Autodesk Inventor part; units mm, degrees
ref_plane "Work Plane1" through (-36, 60, 19) normal (0, -1, 0) x (1, 0, 0)
ref_plane "YZ Plane" through (0, 0, 0) normal (1, 0, 0) x (0, 1, 0)
ref_plane "XZ Plane" through (0, 0, 0) normal (0, 1, 0) x (-1, 0, 0)
sketch "Sketch1" plane through (0, 0, 0) normal (0, 0, 1) x (1, 0, 0)
  arc A0 (36, 0) -> (-36, 0) centre (0, 0) ccw
  arc A1 (27, 0) -> (-27, 0) centre (0, 0) ccw
  line L0 (-36, 0) -> (-27, 0)
  line L1 (27, 0) -> (36, 0)
  dimension "d0" = 72
  dimension "d1" = 54
  dimension "d2" = 27
  dimension "d3" = 36
extrude "Extrusion1" add sketch "Sketch1" along normal mid plane 38
ref_plane "Work Plane1" through (-36, 60, 19) normal (0, -1, 0) x (1, 0, 0)
sketch "Sketch2" plane through (-36, 60, 19) normal (0, -1, 0) x (1, 0, 0)
  line L0 (9, 0) -> (63, 0)
  line L1 (0, -38) -> (0, 0)
  line L2 (-2, -19) -> (74, -19) construction
  line L3 (-2, -31) -> (74, -31)
  line L4 (74, -7) -> (-2, -7)
  arc A0 (-2, -7) -> (-2, -31) centre (-2, -19) ccw
  arc A1 (74, -31) -> (74, -7) centre (74, -19) ccw
  point P0 (36, -19)
  point P1 (36, -19)
  point P2 (36, 0)
  point P3 (-14, -19)
  point P4 (0, -19)
  dimension "d7" = 76
  dimension "d8" = 12
extrude "Extrusion2" add sketch "Sketch2" along normal up to surface (60 mm away)
sketch "Sketch3" plane through (0, 0, 12) normal (0, 0, 1) x (1, 0, 0)
  arc A0 (27, 0) -> (-27, 0) centre (0, 0) ccw
  line L0 (-27, 0) -> (27, 0)
extrude "Extrusion3" cut sketch "Sketch3" against normal through all
sketch "Sketch4" plane through (0, 0, 0) normal (0, 0, 1) x (1, 0, 0)
  arc A0 (27, 0) -> (-27, 0) centre (0, 0) ccw
  line L0 (38, 60) -> (-38, 60)
  line L1 (-50, 60) -> (-50, 0)
  line L2 (-50, 60) -> (-50, 0)
  line L3 (-50, 60) -> (-38, 60)
  line L4 (-50, 40) -> (-24.8, 60)
  line L5 (-50, 40) -> (-50, 60)
  line L6 (0, 0) -> (0, 60) construction
  line L7 (-38, 60) -> (38, 60)
  line L8 (50, 60) -> (50, 0)
  line L9 (50, 60) -> (38, 60)
  line L10 (50, 40) -> (24.8, 60)
  point P0 (24.8, 60)
  point P1 (50, 40)
  point P2 (-50, 40)
  dimension "d13" = 20
  dimension "d14" = 25.2
extrude "Extrusion4" cut sketch "Sketch4" along normal through all both and the other way through all
fillet "Fillet1" radius 10 2 edges at (24.8, 60, 0) (-24.8, 60, 0)
sketch "Sketch5" plane through (-36, 0, 19) normal (0, -1, 0) x (1, 0, 0)
  arc A0 (-2, -7) -> (-2, -31) centre (-2, -19) ccw
  point P0 (36, -19)
  point P1 (0, -31)
  point P2 (0, -7)
hole "Hole1" at (-38, 0, 0) direction (0, 1, 0) diameter 10 end through all
sketch "Sketch6" plane through (27, 0, -19) normal (0, -1, 0) x (1, 0, 0)
  arc A0 (11, 7) -> (11, 31) centre (11, 19) ccw
  point P0 (-27, 19)
  point P1 (9, 31)
  point P2 (9, 7)
hole "Hole2" at (38, 0, 0) direction (0, 1, 0) diameter 10 end through all
sketch "Sketch7" plane through (-36, 60, 19) normal (0, 1, 0) x (1, 0, 0)
  circle A0 centre (-2, 19) radius 5
  circle A1 centre (74, 19) radius 5
  point P0 (36, 19)
hole "Hole3" at (-38, 60, 0) at (38, 60, 0) direction (0, -1, 0) diameter 10 end through all counterbore diameter 19 counterbore depth 25
fillet "Fillet2" radius 3 2 edges at (0, 36, -12) (0, 36, 12)
equation "\"d23\" = Thickness"
equation "\"BendRadius\" = Thickness"
equation "\"BendReliefWidth\" = Thickness"
equation "\"BendReliefDepth\" = 0.5 * Thickness"
equation "\"CornerReliefSize\" = 4 * Thickness"
equation "\"MinimumRemnant\" = 2 * Thickness"
equation "\"TransitionRadius\" = BendRadius"
equation "\"JacobiRadiusSize\" = BendRadius"
equation "\"GapSize\" = Thickness"
properties part number "Part 4 Connecting rods cap" material "Stainless Steel"
Geometry check sheet. Reference: the model listing, model coordinates, mm. A direction names the side the tool comes from. Give positions to 0.01 mm unless a question says otherwise; leave off trailing zeros. Loops run counter-clockwise (first coordinate to the right, second up) from the corner with the lowest first, then second, coordinate; pieces in that order, holes last. Notation, with made-up numbers: M 4,5 L 58,5 A30 cw 58,32 Z; hole C 70,67.25 d1. An arc over 180 degrees is marked long. Answer as a JSON object with one key per item and string values. Group by question number.
Item 1: Sectioned sample at B-B on y = 25.5. Give the number of separate pieces and of enclosed holes in the cut face, plus the area to 3 significant figures.
Item 2: Mould release check, pull along Z, two halves, no side actions. Record for faces 1 (the flat face through (42, 35, 4)), 2 (the cylindrical face through (-28.726, 43.436, -2.059)), 3 (the flat face through (-1, 46, -12)), 4 (the flat face through (-1, 30, 19)): pulls with the +Z half, pulls with the -Z half, needs draft (parallel to the pull), parting line crosses it, or undercut.
Item 3: Sectioned sample at D-D on z = 6. Record the boundary of the cut face in (x, y), plus the area to 3 significant figures.
Item 4: Sectioned sample at A-A on z = 0. Record the boundary of the cut face in (x, y), plus the area to 3 significant figures.
Item 5: Gauge pin test, flat ends, axial feed: pin 1 (5 mm diameter, centred on x = -7, y = 40, fed in from -Z); pin 2 (21 mm diameter, centred on x = -37, z = -4.5, fed in from +Y); pin 3 (16 mm diameter, centred on x = -38, z = 0, fed in from +Y); pin 4 (12 mm diameter, centred on x = 38, z = -0.5, fed in from -Y). Record the tip position at first contact, or that the pin passes through.
Item 6: Sectioned sample at C-C on y = 52.5. Record the boundary of the cut face in (x, z).
Item 7: Material ranges on L1, parallel to X at y = 28, z = 0; L2, parallel to X at y = 8, z = 0; L3, parallel to X at y = 18.5, z = 4.5, recorded low to high.
Item 8: Access from +Z, -Z, +X, -X, +Y, -Y to the whole of each face (thin tool, end or side, straight path). Record for faces 5 (the cylindrical face through (-0.79, 35.99, -17.01)), 6 (the flat face through (-1, 30, -19)), 7 (the cylindrical face through (-0.79, 35.99, 16.96)), 8 (the cylindrical face through (28.58, 43.44, -1.24)).
Findings below:
{
 "1": {"separate pieces": "2", "enclosed holes": "2", "area": "2,170 mm2"},
 "2": {"face 1": "undercut", "face 2": "undercut", "face 3": "pulls with the -Z half", "face 4": "pulls with the +Z half"},
 "3": {"outline": "M -48.39,0 L -27,0 A27 cw 27,0 L 48.39,0 L 48.39,41.28 L 45.37,43.68 L 45.37,35 L 30.63,35 L 30.63,55.37 L 27.53,57.83 A10 ccw 21.31,60 L -21.31,60 A10 ccw -27.53,57.83 L -30.63,55.37 L -30.63,35 L -45.37,35 L -45.37,43.68 L -48.39,41.28 Z", "area": "3,790 mm2"},
 "4": {"outline": "M -50,0 L -43,0 L -43,35 L -47.5,35 L -47.5,41.98 L -50,40 Z; M -33,0 L -27,0 A27 cw 27,0 L 33,0 L 33,35 L 28.5,35 L 28.5,57.06 L 27.53,57.83 A10 ccw 21.31,60 L -21.31,60 A10 ccw -27.53,57.83 L -28.5,57.06 L -28.5,35 L -33,35 Z; M 43,0 L 50,0 L 50,40 L 47.5,41.98 L 47.5,35 L 43,35 Z", "area": "3,100 mm2"},
 "5": {"pin 1": "z = -12.14", "pin 2": "y = 58.55", "pin 3": "y = 35", "pin 4": "y = 0"},
 "6": {"outline": "M -34.25,-12 L 34.25,-12 L 34.25,-8.73 A9.5 cw 34.25,8.73 L 34.25,12 L -34.25,12 L -34.25,8.73 A9.5 cw -34.25,-8.73 Z"},
 "7": {"L1": "-50 to -43, -33 to 33, 43 to 50", "L2": "-50 to -43, -33 to -25.79, 25.79 to 33, 43 to 50", "L3": "-49.12 to -40.18, -35.82 to -19.67, 19.67 to 35.82, 40.18 to 49.12"},
 "8": {"face 5": "-Z, +Y", "face 6": "-Z, +X, -X, +Y, -Y", "face 7": "+Z, +Y", "face 8": "+Y"}
}
